Could you check a few things on this model? Use its own coordinates, in mm. A direction names the side the tool comes from. Give positions to 0.01 mm unless a question says otherwise; leave off trailing zeros. Order: outer loops, then holes, each group sorted by start corner. A loop starts at its lowest first (then second) coordinate and runs counter-clockwise, first axis right, second up. Notation, with made-up numbers: (39.25, -22.75) -> (82.25, -22.75) arc R25 ccw to (82.25, 9.25) -> close; hole circle Ø6 at (2.5, -38). An arc over 180 degrees is marked (long way). Answer as CSV lines item,"result". Start each with the question number.
(1) Will these pins go through, and if not, where does the flat tip stop? pin 1 Ø2 at (x, z) = (11, 1.5) entering from +Y; pin 2 Ø1 at (y, z) = (-1, 2.5) entering from -X.
(2) I need wall thicknesses on L1, parallel to X at y = -0.25, z = 0.5; L2, parallel to Z at x = 28, y = 2.75; L3, parallel to X at y = 0.5, z = 5.5. Which ranges of each line are inside material? Lowest first, please.
(3) I want a section at B-B (x = 31.5). Please give me the cut outline in (y, z).
(4) On a 3-axis mill with a long thin cutter (end or side, diameter ignored), from which of +Z, -Z, +X, -X, +Y, -Y can I reach the whole of each face in a straight line? I mean faces 4 (the face through (20, 0, 6)), 5 (the face through (0.521, -0.655, 3.295)). Say none if no direction works.
(5) We'd pull the mould along Y, two halves only. Please class faces 1 (the face through (40, 0, 3)), 2 (the face through (30.14, 0.218, 5.094)), 3 (the face through (21.759, 0.946, 0.145)): released by +Y, released by -Y, zero draft, split by the parting line, or undercut.
(6) I want a section at A-A (x = 17.5). Please give me the cut outline in (y, z), plus the area to 3 significant figures.
```python
from build123d import *

# Parameters (mm, degrees)
F0_W     = 40
F0_H     = 3.15
F2_SIZE  = 3
F4_DEPTH = 20


with BuildPart() as f1:
    # F0 (on Front) → F1 (revolve)
    with BuildSketch(Plane.XZ):
        with Locations((20, 1.575)):
            Rectangle(F0_W, F0_H)
    revolve(axis=Axis((20, 0, 3.15), (1, 0, 0)))

    # F2
    f2_edges = [f1.edges().sort_by_distance(p)[0] for p in [
        (0, 0, 6.3),
    ]]
    chamfer(f2_edges, length=F2_SIZE)

    # F3 (on face) → F4 (cut)
    with BuildSketch(Plane.YZ.offset(40)):
        Polygon((2.034494, 6.619173), (-1.549196, 6.880851), (-1.549196, 5.222723), (2.034494, 4.961044), align=None)
    extrude(amount=-F4_DEPTH, mode=Mode.SUBTRACT)


solid = f1.part
```
Final values:
1,pin 1,"y = 3.08"
1,pin 2,"x = 0.54"
2,L1,"2.51 to 40"
2,L2,"1.61 to 4.69"
2,L3,"2.25 to 20"
3,outline,"(-1.55, 5.22) -> (-1.55, 5.89) arc R3.15 ccw (long way) to (2.03, 5.55) -> (2.03, 4.96) -> close"
4,face 4,"+Z, +X"
4,face 5,"-X"
5,face 1,"zero draft"
5,face 2,"undercut"
5,face 3,"split by the parting line"
6,outline,"circle Ø6.3 at (0, 3.15)"
6,area,"31.2 mm²"
